Could you check a few things on this drawing? It's one solid part, dimensions in mm from its lowest x, y, z. Give positions to 0.01 mm unless a question says otherwise; leave off trailing zeros. Loops run counter-clockwise (first coordinate to the right, second up) from the corner with the lowest first, then second, coordinate; pieces in that order, holes last. Notation, with made-up numbers: M -21.5,-37.75 L 17.5,-37.75 A17 cw 17.5,-31.75 Z; hole C -24,5 d8. An arc over 180 degrees is marked long. Answer as a JSON object with one key per item and string values.
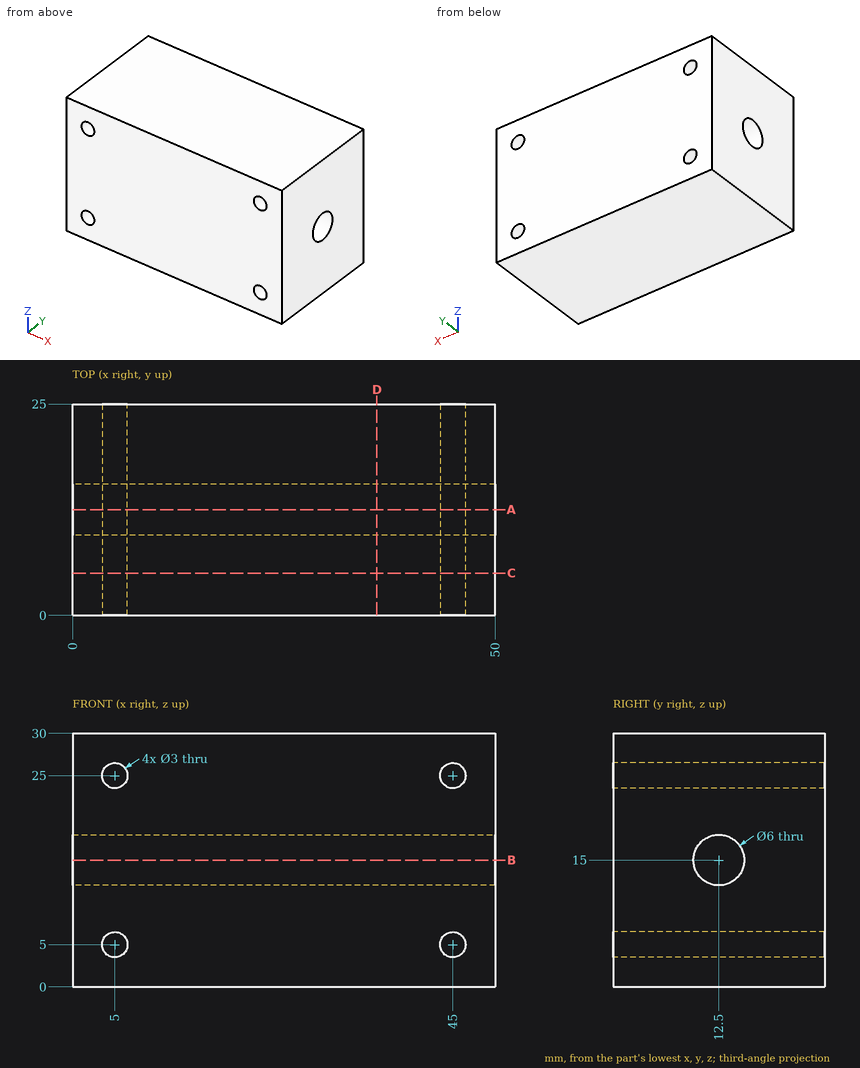
1) Suppose I cut it at D-D, the plane x = 36. Write out the boundary of the cut face in (y, z), and give its area (3 significant figures).
Answer list:
{"outline": "M 0,0 L 25,0 L 25,30 L 0,30 Z; hole C 12.5,15 d6", "area": "722 mm^2"}
2) Please list where these lines run through material, in increasing order: line 1 along X through (y, z) = (9.75, 25); line 2 along X through (y, z) = (12.75, 3.75); line 3 along Z through (x, y) = (44.5, 9). Write a range as from..to.
Answer list:
{"line 1": "0..3.5, 6.5..43.5, 46.5..50", "line 2": "0..4.17, 5.83..44.17, 45.83..50", "line 3": "0..3.59, 6.41..23.59, 26.41..30"}
3) Will these pins go through, and if not, where does the flat tip stop? pin 1 Ø3.5 at (x, z) = (45, 25) entering from +Y; pin 2 Ø5.5 at (y, z) = (12.5, 15) entering from -X.
Answer list:
{"pin 1": "y = 25", "pin 2": "through"}
4) Suppose I cut it at A-A, the plane y = 12.5. Write out the boundary of the cut face in (x, z).
Answer list:
{"outline": "M 0,0 L 50,0 L 50,12 L 0,12 Z; M 0,18 L 50,18 L 50,30 L 0,30 Z; hole C 5,5 d3; hole C 5,25 d3; hole C 45,5 d3; hole C 45,25 d3"}
5) Suppose I cut it at B-B, the plane z = 15. Write out the boundary of the cut face in (x, y).
Answer list:
{"outline": "M 0,0 L 50,0 L 50,9.5 L 0,9.5 Z; M 0,15.5 L 50,15.5 L 50,25 L 0,25 Z"}
6) Suppose I cut it at C-C, the plane y = 5. Write out the boundary of the cut face in (x, z).
Answer list:
{"outline": "M 0,0 L 50,0 L 50,30 L 0,30 Z; hole C 5,5 d3; hole C 5,25 d3; hole C 45,5 d3; hole C 45,25 d3"}
